Verification items for the finished model (mm, model axes). Face numbers are marked on the shaded views. Give positions to 0.01 mm unless a question says otherwise; leave off trailing zeros. Write each loop counter-clockwise with the first axis right and the second up, starting at its lowest first coordinate (ties: lowest second). Pieces come first, ordered by that corner, then holes. Notation, with made-up numbers: M 56,39 L 79,39 A28 ccw 79,59 Z; hole C 19.25,25.5 d7. An arc over 180 degrees is marked long. Answer as a JSON object with one key per item and string values.
```python
from build123d import *

# Parameters (mm, degrees)
F1_DEPTH = 100
F2_W     = 2.322293818
F2_H     = 11.1691281199
F3_DEPTH = 26.5967446956
F4_R     = 2.25
F5_DEPTH = 5


with BuildPart() as f1:
    # F0 (on Top) → F1 (new body)
    with BuildSketch(Plane.XY):
        Polygon((13.0718629807, 13.9992671447), (-13.5238817149, 13.9992671447), (-13.5238817149, 7.3329959996), (-11.4936745146, 7.3329959996), (13.0718629807, 7.3329959996), align=None)
        with BuildLine():
            ThreePointArc((13.0718629807, 13.9992671447), (-0.2260093671, 19.4983686983), (-13.5238817149, 13.9992671447))
            Line((-13.5238817149, 13.9992671447), (13.0718629807, 13.9992671447))
        make_face()
        Polygon((-11.4936745146, 7.3329959996), (-13.5238817149, 7.3329959996), (-8.7926732376, -19.7865962982), (-6.8224309887, -19.4428733275), align=None)
    extrude(amount=F1_DEPTH)

    # F2 (on face) → F3 (cut, through all)
    with BuildSketch(Plane(origin=(-13.5238817149, 0, 0), x_dir=(0, -1, 0), z_dir=(-1, 0, 0))):
        with Locations((-10.6661058962, 91.6783995926)):
            Rectangle(F2_W, F2_H)
        with Locations((-10.6661058962, 70.7783995926)):
            Rectangle(F2_W, F2_H)
        with Locations((-10.6661058962, 49.8783995926)):
            Rectangle(F2_W, F2_H)
        with Locations((-10.6661058962, 28.9783995926)):
            Rectangle(F2_W, F2_H)
        with Locations((-10.6661058962, 8.0783995926)):
            Rectangle(F2_W, F2_H)
    extrude(amount=-F3_DEPTH, mode=Mode.SUBTRACT)

    # F4 (on face) → F5 (cut)
    with BuildSketch(Plane(origin=(-11.8829269994, -2.073062321, 0), x_dir=(0.1718614854, -0.9851211245, 0), z_dir=(-0.9851211245, -0.1718614854, 0))):
        with Locations((2.8274371289, 93.9120426774)):
            Circle(F4_R)
        with Locations((2.8274371289, 4.9835015088)):
            Circle(F4_R)
        Polygon((14.1747677699, 69.6047618985), (14.6328052506, 96.599586308), (-6.3302433118, 82.4077576399), align=None)
        Polygon((-5.5054374928, 51.6755245626), (14.6328052506, 64.7412315011), (-5.5054374928, 77.3152230515), align=None)
        Polygon((13.5203069012, 34.5346203232), (14.6328052506, 60.2121762931), (-5.6320335211, 46.4930304839), align=None)
        Polygon((-5.4043177298, 19.6944773197), (13.6406598613, 30.2205141634), (-5.4043177298, 42.1118887167), align=None)
        Polygon((14.6328052506, 5.2338945679), (14.6328052506, 26.8068239093), (-4.4452575967, 15.9530360252), align=None)
    extrude(amount=-F5_DEPTH, mode=Mode.SUBTRACT)


solid = f1.part
```
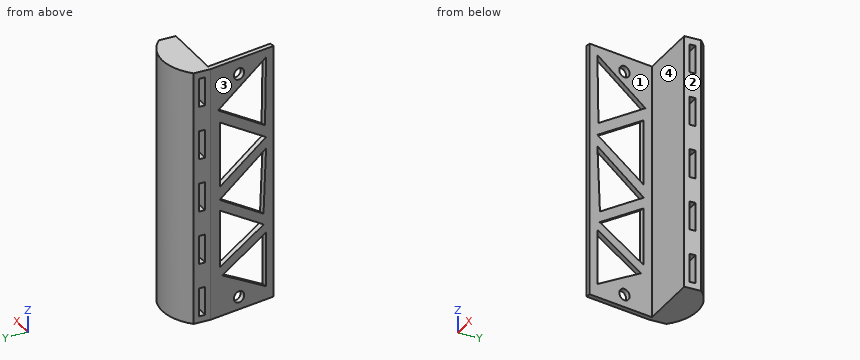
1) Section check B-B on x = -3.25. Record the boundary of the cut face in (y, z).
Completed:
{"outline": "M 7.33,0 L 19.25,0 L 19.25,100 L 7.33,100 Z; hole M 9.5,2.49 L 11.83,2.49 L 11.83,13.66 L 9.5,13.66 Z; hole M 9.5,23.39 L 11.83,23.39 L 11.83,34.56 L 9.5,34.56 Z; hole M 9.5,44.29 L 11.83,44.29 L 11.83,55.46 L 9.5,55.46 Z; hole M 9.5,65.19 L 11.83,65.19 L 11.83,76.36 L 9.5,76.36 Z; hole M 9.5,86.09 L 11.83,86.09 L 11.83,97.26 L 9.5,97.26 Z"}
2) Section check A-A on z = 90.5. Record the boundary of the cut face in (x, y).
Completed:
{"outline": "M -13.52,7.33 L -10.92,-7.61 L -8.95,-7.27 L -11.49,7.33 L 13.07,7.33 L 13.07,9.5 L -13.52,9.5 Z; M -13.52,11.83 L 13.07,11.83 L 13.07,14 A18.83 ccw -13.52,14 Z; M -9.39,-16.39 L -8.79,-19.79 L -6.82,-19.44 L -7.42,-16.04 Z"}
3) Go/stop test with flat-tipped pins: pin 1 (5 mm diameter, centred on x = -8, z = 57, fed in from +Y); pin 2 (3.5 mm diameter, centred on x = 2, z = 89, fed in from -Y); pin 3 (5.5 mm diameter, centred on x = -6.5, z = 68.5, fed in from +Y). Record where each tip stops, or that it passes through.
Completed:
{"pin 1": "stops at y = 18.74", "pin 2": "stops at y = 7.33", "pin 3": "stops at y = 19.17"}
4) Release check for a two-part mould opening along Y. For the marked faces 1, 2, 3 and 4 record: pulls with the +Y half, pulls with the -Y half, needs draft (parallel to the pull), parting line crosses it, or undercut.
Completed:
{"face 1": "undercut", "face 2": "needs draft", "face 3": "pulls with the -Y half", "face 4": "undercut"}
5) Section check D-D on z = 11.5. Record the boundary of the cut face in (x, y).
Completed:
{"outline": "M -13.52,7.33 L -11.28,-5.5 L -9.31,-5.16 L -11.49,7.33 L 13.07,7.33 L 13.07,9.5 L -13.52,9.5 Z; M -13.52,11.83 L 13.07,11.83 L 13.07,14 A18.83 ccw -13.52,14 Z; M -9.37,-16.49 L -8.79,-19.79 L -6.82,-19.44 L -7.4,-16.14 Z"}
6) Thickness scan on L1, parallel to Y at x = -8.75, z = 50; L2, parallel to Y at x = 0.5, z = 31; L3, parallel to Z at x = -10.5, y = 0.5. Record the ranges inside material, lowest first.
Completed:
{"L1": "y = -19.78 to -15.93, 7.33 to 9.5, 11.83 to 17.46", "L2": "y = 7.33 to 9.5, 11.83 to 19.48", "L3": "z = 0 to 14.75, 17.18 to 21.41, 40.17 to 44.41, 48.75 to 53.76, 75.31 to 79.89, 85.14 to 100"}
7) Section check C-C on z = 43. Record the boundary of the cut face in (x, y).
Completed:
{"outline": "M -13.52,7.33 L -11.89,-2.04 L -9.92,-1.69 L -11.49,7.33 L 13.07,7.33 L 13.07,14 A18.83 ccw -13.52,14 Z; M -9.5,-15.75 L -8.79,-19.79 L -6.82,-19.44 L -7.53,-15.41 Z"}
